Design review of the part shown in the three views and the two pictorial views. Dimensions are in mm from the part's minimum x, y and z. A direction names the side the tool comes from. Coordinates: 2 decimals unless noted, no trailing zeros. Loops run counter-clockwise (first coordinate to the right, second up) from the corner with the lowest first, then second, coordinate; pieces in that order, holes last. Notation, with made-up numbers: (-29.75, -3.5) -> (0.25, -3.5) arc R22 ccw to (0.25, 4.5) -> close; hole circle Ø2 at (6.25, 28.5). An arc over 180 degrees is marked (long way). Answer in a Markdown table with one row per item.
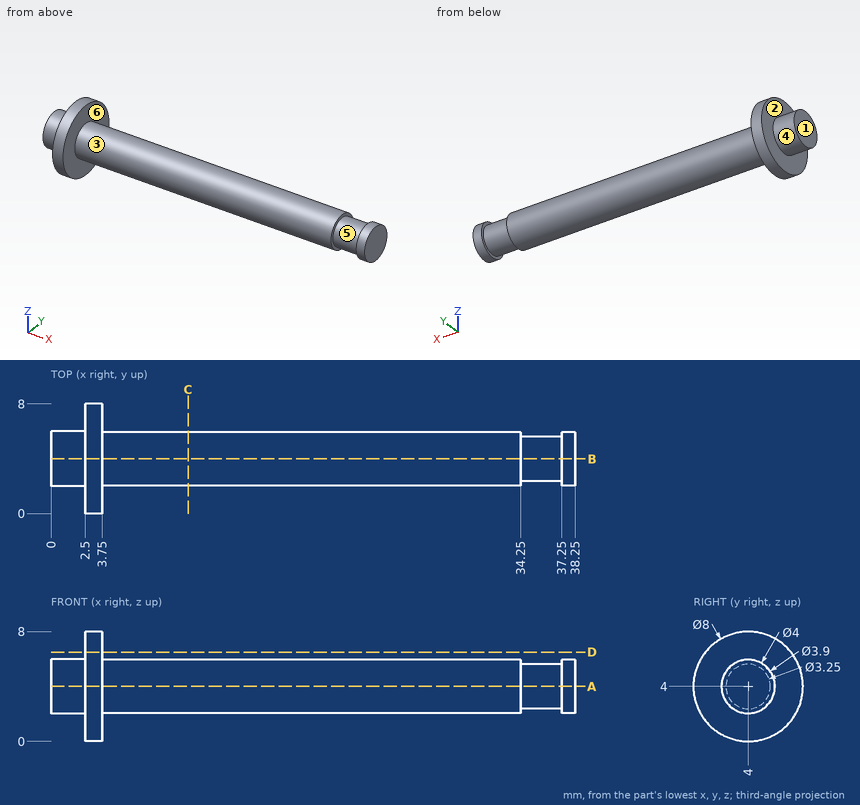
Item 1: For L1, parallel to X at y = 4.25, z = 2.25; L2, parallel to X at y = 5, z = 6; L3, parallel to Z at x = 15, y = 4, list the stretches that pass through material, from the lowest coordinate up.
Worked answers:
| item | result |
|---|---|
| L1 | 0 to 34.25, 37.25 to 38.25 |
| L2 | 2.5 to 3.75 |
| L3 | 2.05 to 5.95 |
Item 2: Take a section at C-C, the plane x = 10. State the section outline as (y, z) points, and give its area (3 significant figures).
Worked answers:
| item | result |
|---|---|
| outline | circle Ø3.9 at (4, 4) |
| area | 11.9 mm² |
Item 3: Take a section at D-D, the plane z = 6.5. State the section outline as (x, y) points, and give its area (3 significant figures).
Worked answers:
| item | result |
|---|---|
| outline | (2.5, 0.88) -> (3.75, 0.88) -> (3.75, 7.12) -> (2.5, 7.12) -> close |
| area | 7.81 mm² |
Item 4: Insertion check: pin 1 (4 mm diameter, centred on x = 6.5, y = 4.5, fed in from -Z); pin 2 (2 mm diameter, centred on y = 4, z = 3, fed in from -X); pin 3 (2 mm diameter, centred on x = 14, y = 6, fed in from -Z). Each pin has a flat end and moves straight along its axis. Give the tip position at first contact, or say it passes through.
Worked answers:
| item | result |
|---|---|
| pin 1 | z = 2.05 |
| pin 2 | x = 0 |
| pin 3 | z = 2.33 |
Item 5: For the marked faces 1, 2 and 3, list the 3-axis set-ups (+Z, -Z, +X, -X, +Y, -Y) from which the entire face can be reached by the end or side of a thin tool; tool diameter is ignored.
Worked answers:
| item | result |
|---|---|
| face 1 | +Z, -Z, -X, +Y, -Y |
| face 2 | -X |
| face 3 | +X |
Item 6: The part is to be moulded in two halves that separate along X. For the marked faces 4, 5 and 6, say which applies: +X half, -X half, draft (parallel to the pull), parting line (faces both ways), or undercut.
Worked answers:
| item | result |
|---|---|
| face 4 | draft |
| face 5 | undercut |
| face 6 | +X half |
Item 7: Take a section at A-A, the plane z = 4. State the section outline as (x, y) points (3 decimals).
Worked answers:
| item | result |
|---|---|
| outline | (0, 2) -> (2.5, 2) -> (2.5, 0) -> (3.75, 0) -> (3.75, 2.05) -> (34.25, 2.05) -> (34.25, 2.375) -> (37.25, 2.375) -> (37.25, 2.05) -> (38.25, 2.05) -> (38.25, 5.95) -> (37.25, 5.95) -> (37.25, 5.625) -> (34.25, 5.625) -> (34.25, 5.95) -> (3.75, 5.95) -> (3.75, 8) -> (2.5, 8) -> (2.5, 6) -> (0, 6) -> close |
